from build123d import *

# Parameters (mm, degrees)
SKETCH_1_R      = 1.525
EXTRUDE_1_DEPTH = 4.5
SKETCH_2_W      = 5
SKETCH_2_H      = 3
EXTRUDE_2_DEPTH = 4
FILLET_1_R      = 3.5
FILLET_3_R      = 1.5
FILLET_4_R      = 5
FILLET_5_R      = 2


with BuildPart() as part:
    # 草图1 → 凸台-拉伸1 (new body)
    with BuildSketch(Plane(origin=(0, 0, 0), x_dir=(1, 0, 0), z_dir=(0, 1, 0))):
        Polygon((3.5, -3.5), (3.5, 18), (-3.5, 18), (-3.5, 6.5), (-8.5, 6.5), (-8.5, 3.5), (-28.5, 3.5), (-28.5, -3.5), (-13, -3.5), (-13, -8.5), (-7.55, -8.5), (-1.95, -8.5), (-1.95, -3.5), align=None)
        with Locations(Location((0, 0, 0), (0, 0, 270))):
            Circle(SKETCH_1_R, mode=Mode.SUBTRACT)
    extrude(amount=EXTRUDE_1_DEPTH)

    # 草图2 → 凸台-拉伸2 (add)
    with BuildSketch(Plane(origin=(0, 0, 0), x_dir=(1, 0, 0), z_dir=(0, 1, 0))):
        with Locations((-6, 5)):
            Rectangle(SKETCH_2_W, SKETCH_2_H)
    extrude(amount=-EXTRUDE_2_DEPTH)

    # 圆角1
    fillet_1_edges = [part.edges().sort_by_distance(p)[0] for p in [
        (3.5, 2.25, -18),
        (-3.5, 2.25, -18),
        (-28.5, 2.25, 3.5),
        (-28.5, 2.25, -3.5),
    ]]
    fillet(fillet_1_edges, radius=FILLET_1_R - 0.0001)  # a hair under: the kernel refuses the full size

    # 圆角3
    fillet_3_edges = [part.edges().sort_by_distance(p)[0] for p in [
        (-8.5, 2.25, -3.5),
        (-8.5, 0.25, -6.5),
        (-3.5, 2.25, -6.5),
    ]]
    fillet(fillet_3_edges, radius=FILLET_3_R - 0.0001)  # a hair under: the kernel refuses the full size

    # 圆角4
    fillet_4_edges = [part.edges().sort_by_distance(p)[0] for p in [
        (-13, 2.25, 8.5),
    ]]
    fillet(fillet_4_edges, radius=FILLET_4_R - 0.0001)  # a hair under: the kernel refuses the full size

    # 圆角5
    fillet_5_edges = [part.edges().sort_by_distance(p)[0] for p in [
        (3.5, 2.25, 3.5),
        (-1.95, 2.25, 3.5),
    ]]
    fillet(fillet_5_edges, radius=FILLET_5_R)


solid = part.part
Can you work these out from the model? Positions are in its coordinate system, mm. A direction names the side the tool comes from. Coordinates: 2 decimals unless noted, no trailing zeros. Order: outer loops, then holes, each group sorted by start corner. A loop starts at its lowest first (then second) coordinate and runs counter-clockwise, first axis right, second up. Notation, with made-up numbers: (88.5, 43) - (102.5, 43) arc R15 cw to (102.5, 65) - close; hole circle Ø4 at (85.5, -7.75). An arc over 180 degrees is marked (long way). Answer as a JSON object with one key per item and string values. Group by question number.
Q1. On a 3-axis mill with a long thin cutter (end or side, diameter ignored), from which of +Z, -Z, +X, -X, +Y, -Y can I reach the whole of each face in a straight line? I mean faces 4 (the face through (1, 2, 3.5)), 5 (the face through (-19, 2, 3.5)), 6 (the face through (-3.5, 2, -11)). Say none if no direction works.
Q2. Will these pins go through, and if not, where does the flat tip stop? P1, Ø1.3, axis at y = 2, z = -11.5, coming from the -X side; P2, Ø0.9, axis at y = 2, z = 7, coming from the +X side; P3, Ø5, axis at x = -0.5, y = -1.5, coming from the -Z side; P4, Ø2, axis at x = -20.5, y = 2.5, coming from the +Z side.
Q3. We'd pull the mould along X, two halves only. Please class faces 1 (the face through (3.5, 2, -6)), 2 (the face through (-0.93, 2.22, -1.21)), 3 (the face through (-11.57, 2.28, 7)): +X half, -X half, draft (parallel to the pull), parting line (faces both ways), or undercut.
Q4. Imagine slicing it at A-A (x = -6). Please give me the cut outline in (y, z), and give its area (3 significant figures).
Q5. Imagine slicing it at C-C (z = -11.5). Please give me the cut outline in (x, y), and give its area (3 significant figures).
Q6. I need wall thicknesses on line 1 (X direction, y = 2.1, z = 0) (3 decimals); line 2 (X direction, y = 3, z = -8.5). Which ranges of each line are inside material? Lowest first, please. Write a range as from..to.
Q7. Imagine slicing it at D-D (x = -11). Please give me the cut outline in (y, z).
Q8. Imagine slicing it at B-B (y = -3.5). Please give me the cut outline in (x, z).
Determined:
{
 "1": {"face 4": "+Z, +X, +Y, -Y", "face 5": "+Z, -X, +Y, -Y", "face 6": "-Z, -X, +Y, -Y"},
 "2": {"P1": "stops at x = -3.5", "P2": "stops at x = -1.95", "P3": "stops at z = -18", "P4": "stops at z = 3.5"},
 "3": {"face 1": "+X half", "face 2": "undercut", "face 3": "-X half"},
 "4": {"outline": "(-4, -6.5) - (4.5, -6.5) - (4.5, 8.5) - (0, 8.5) - (0, -3.5) - (-4, -3.5) - close", "area": "79.5 mm2"},
 "5": {"outline": "(-3.5, 0) - (3.5, 0) - (3.5, 4.5) - (-3.5, 4.5) - close", "area": "31.5 mm2"},
 "6": {"line 1": "x = -28.5..-1.525, 1.525..3.5", "line 2": "x = -3.5..3.5"},
 "7": {"outline": "(0, -3.5) - (4.5, -3.5) - (4.5, 7.5) - (0, 7.5) - close"},
 "8": {"outline": "(-8.5, -5) arc R1.5 ccw to (-7, -6.5) - (-3.5, -6.5) - (-3.5, -3.5) - (-8.5, -3.5) - close"}
}
